from build123d import *

# Parameters (mm, degrees)
BOSS_EXTRUDE1_DEPTH = 3
SKETCH2_R           = 0.75
BOSS_EXTRUDE2_DEPTH = 3
SKETCH3_R           = 2.5
BOSS_EXTRUDE3_DEPTH = 0.5
SKETCH4_R           = 2
BOSS_EXTRUDE4_DEPTH = 2.5


with BuildPart() as part:
    # Sketch1 → Boss-Extrude1 (new body)
    with BuildSketch(Plane(origin=(0, 0, 0), x_dir=(1, 0, 0), z_dir=(0, 1, 0))):
        with BuildLine():
            ThreePointArc((0.59835355, 4.007919609), (0.660413192, 4.106024801), (0.773897857, 4.130463677))
            ThreePointArc((0.773897857, 4.130463677), (0.935108267, 4.096977009), (1.094883149, 4.057200879))
            ThreePointArc((1.094883149, 4.057200879), (1.186525668, 3.985943061), (1.199873226, 3.870626668))
            ThreePointArc((1.199873226, 3.870626668), (1.497913497, 3.110449426), (2.278069066, 3.351394917))
            ThreePointArc((2.278069066, 3.351394917), (2.376549119, 3.412857971), (2.4893989, 3.385637488))
            ThreePointArc((2.4893989, 3.385637488), (2.62011514, 3.285520466), (2.746809119, 3.180359688))
            ThreePointArc((2.746809119, 3.180359688), (2.798458567, 3.076396414), (2.760450393, 2.966708646))
            ThreePointArc((2.760450393, 2.966708646), (2.699146854, 2.152497789), (3.506585066, 2.03108536))
            ThreePointArc((3.506585066, 2.03108536), (3.621980347, 2.043732765), (3.711843962, 1.970244271))
            ThreePointArc((3.711843962, 1.970244271), (3.786176077, 1.823326301), (3.854695856, 1.673609257))
            ThreePointArc((3.854695856, 1.673609257), (3.856122426, 1.557531728), (3.774286506, 1.475197592))
            ThreePointArc((3.774286506, 1.475197592), (3.365781075, 0.768217567), (4.040578887, 0.308494438))
            ThreePointArc((4.040578887, 0.308494438), (4.150033947, 0.269821219), (4.199112803, 0.164620014))
            ThreePointArc((4.199112803, 0.164620014), (4.202338407, 0), (4.199112803, -0.164620014))
            ThreePointArc((4.199112803, -0.164620014), (4.150033947, -0.269821219), (4.040578887, -0.308494438))
            ThreePointArc((4.040578887, -0.308494438), (3.365781075, -0.768217567), (3.774286506, -1.475197592))
            ThreePointArc((3.774286506, -1.475197592), (3.856122426, -1.557531728), (3.854695856, -1.673609257))
            ThreePointArc((3.854695856, -1.673609257), (3.786176077, -1.823326301), (3.711843962, -1.970244271))
            ThreePointArc((3.711843962, -1.970244271), (3.621980347, -2.043732765), (3.506585066, -2.03108536))
            ThreePointArc((3.506585066, -2.03108536), (2.699146854, -2.152497789), (2.760450393, -2.966708646))
            ThreePointArc((2.760450393, -2.966708646), (2.798458567, -3.076396414), (2.746809119, -3.180359688))
            ThreePointArc((2.746809119, -3.180359688), (2.62011514, -3.285520466), (2.4893989, -3.385637488))
            ThreePointArc((2.4893989, -3.385637488), (2.376549119, -3.412857971), (2.278069066, -3.351394917))
            ThreePointArc((2.278069066, -3.351394917), (1.497913497, -3.110449426), (1.199873226, -3.870626668))
            ThreePointArc((1.199873226, -3.870626668), (1.186525668, -3.985943061), (1.094883149, -4.057200879))
            ThreePointArc((1.094883149, -4.057200879), (0.935108267, -4.096977009), (0.773897857, -4.130463677))
            ThreePointArc((0.773897857, -4.130463677), (0.660413192, -4.106024801), (0.59835355, -4.007919609))
            ThreePointArc((0.59835355, -4.007919609), (0, -3.452338407), (-0.59835355, -4.007919609))
            ThreePointArc((-0.59835355, -4.007919609), (-0.660413192, -4.106024801), (-0.773897857, -4.130463677))
            ThreePointArc((-0.773897857, -4.130463677), (-0.935108267, -4.096977009), (-1.094883149, -4.057200879))
            ThreePointArc((-1.094883149, -4.057200879), (-1.186525668, -3.985943061), (-1.199873226, -3.870626668))
            ThreePointArc((-1.199873226, -3.870626668), (-1.497913497, -3.110449426), (-2.278069066, -3.351394917))
            ThreePointArc((-2.278069066, -3.351394917), (-2.376549119, -3.412857971), (-2.4893989, -3.385637488))
            ThreePointArc((-2.4893989, -3.385637488), (-2.62011514, -3.285520466), (-2.746809119, -3.180359688))
            ThreePointArc((-2.746809119, -3.180359688), (-2.798458567, -3.076396414), (-2.760450393, -2.966708646))
            ThreePointArc((-2.760450393, -2.966708646), (-2.699146854, -2.152497789), (-3.506585066, -2.03108536))
            ThreePointArc((-3.506585066, -2.03108536), (-3.621980347, -2.043732765), (-3.711843962, -1.970244271))
            ThreePointArc((-3.711843962, -1.970244271), (-3.786176077, -1.823326301), (-3.854695856, -1.673609257))
            ThreePointArc((-3.854695856, -1.673609257), (-3.856122426, -1.557531728), (-3.774286506, -1.475197592))
            ThreePointArc((-3.774286506, -1.475197592), (-3.365781075, -0.768217567), (-4.040578887, -0.308494438))
            ThreePointArc((-4.040578887, -0.308494438), (-4.150033947, -0.269821219), (-4.199112803, -0.164620014))
            ThreePointArc((-4.199112803, -0.164620014), (-4.202338407, 0), (-4.199112803, 0.164620014))
            ThreePointArc((-4.199112803, 0.164620014), (-4.150033947, 0.269821219), (-4.040578887, 0.308494438))
            ThreePointArc((-4.040578887, 0.308494438), (-3.365781075, 0.768217567), (-3.774286506, 1.475197592))
            ThreePointArc((-3.774286506, 1.475197592), (-3.856122426, 1.557531728), (-3.854695856, 1.673609257))
            ThreePointArc((-3.854695856, 1.673609257), (-3.786176077, 1.823326301), (-3.711843962, 1.970244271))
            ThreePointArc((-3.711843962, 1.970244271), (-3.621980347, 2.043732765), (-3.506585066, 2.03108536))
            ThreePointArc((-3.506585066, 2.03108536), (-2.699146854, 2.152497789), (-2.760450393, 2.966708646))
            ThreePointArc((-2.760450393, 2.966708646), (-2.798458567, 3.076396414), (-2.746809119, 3.180359688))
            ThreePointArc((-2.746809119, 3.180359688), (-2.62011514, 3.285520466), (-2.4893989, 3.385637488))
            ThreePointArc((-2.4893989, 3.385637488), (-2.376549119, 3.412857971), (-2.278069066, 3.351394917))
            ThreePointArc((-2.278069066, 3.351394917), (-1.497913497, 3.110449426), (-1.199873226, 3.870626668))
            ThreePointArc((-1.199873226, 3.870626668), (-1.186525668, 3.985943061), (-1.094883149, 4.057200879))
            ThreePointArc((-1.094883149, 4.057200879), (-0.935108267, 4.096977009), (-0.773897857, 4.130463677))
            ThreePointArc((-0.773897857, 4.130463677), (-0.660413192, 4.106024801), (-0.59835355, 4.007919609))
            ThreePointArc((-0.59835355, 4.007919609), (0, 3.452338407), (0.59835355, 4.007919609))
        make_face()
    extrude(amount=BOSS_EXTRUDE1_DEPTH)

    # Sketch2 → Boss-Extrude2 (add)
    with BuildSketch(Plane(origin=(0, 0, 0), x_dir=(-1, 0, 0), z_dir=(0, -1, 0))):
        with Locations(Location((0, 0, 0), (0, 0, 270))):
            Circle(SKETCH2_R)
    extrude(amount=BOSS_EXTRUDE2_DEPTH)

    # Sketch3 → Boss-Extrude3 (add)
    with BuildSketch(Plane(origin=(0, 3, 0), x_dir=(1, 0, 0), z_dir=(0, 1, 0))):
        with Locations(Location((0, 0, 0), (0, 0, 270))):
            Circle(SKETCH3_R)
    extrude(amount=BOSS_EXTRUDE3_DEPTH)

    # Sketch4 → Boss-Extrude4 (add)
    with BuildSketch(Plane(origin=(0, 3.5, 0), x_dir=(1, 0, 0), z_dir=(0, 1, 0))):
        with Locations(Location((0, 0, 0), (0, 0, 270))):
            Circle(SKETCH4_R)
    extrude(amount=BOSS_EXTRUDE4_DEPTH)


solid = part.part
Could you check a few things on this model? Use its own coordinates, in mm. A direction names the side the tool comes from. Coordinates: 2 decimals unless noted, no trailing zeros. Write each loop counter-clockwise with the first axis right and the second up, starting at its lowest first coordinate (ties: lowest second). Pieces come first, ordered by that corner, then holes. Notation, with made-up numbers: (80.5, 50) - (104.5, 50) arc R21 ccw to (104.5, 73) - close; hole circle Ø6 at (-27, -11). An arc over 180 degrees is marked (long way). Put each result on its own line as item: value. Start each with the question number.
Q1. Please list where these lines run through material, in increasing order: L1, parallel to Y at x = -0.5, z = -3.5; L2, parallel to X at y = -1.5, z = 0; L3, parallel to X at y = 1.75, z = 2.
Q2. I'm going to push flat-ended pins straight in: P1, Ø3, axis at x = 3, z = 3.5, coming from the +Y side; P2, Ø3, axis at y = 5, z = 3, coming from the +X side; P3, Ø2, axis at x = -3.5, y = -0.5, coming from the +Z side. Where does each tip first touch, or does it pass through?
Q3. Thinking about a two-plate mould opening in Z: for faces 4 (the cylindrical face through (-3.369, 1.479, -0.756)), 5 (the flat face through (-2, 3, 2)), 6 (the cylindrical face through (-0.013, 1.479, -3.452)), which applies, pulls with the +Z half, pulls with the -Z half, needs draft (parallel to the pull), parting line crosses it, or undercut?
Q4. I want a section at B-B on x = 0. Write out the boundary of the cut face in (y, z).
Q5. I want a section at C-C on z = 3.75. Write out the boundary of the cut face in (x, y), plus the area to 3 significant figures.
Q6. Which directions (+Z, -Z, +X, -X, +Y, -Y) give clear straight access to the entire face, cutting with the end or side of a thin tool? Please do faces 1 (the flat face through (0, 6, 0)), 2 (the cylindrical face through (-2.44, 3.25, -0.54)), 3 (the cylindrical face through (-0.225, -1.479, 0.715)).
Q7. I want a section at A-A on z = 0. Write out the boundary of the cut face in (x, y).
Q8. I want a section at D-D on y = 5. Write out the boundary of the cut face in (x, z).
Checks:
1. L1: 0 to 3
1. L2: -0.75 to 0.75
1. L3: -3.69 to -3.46, -2.88 to 2.88, 3.46 to 3.69
2. P1: y = 3
2. P2: x = 1.32
2. P3: z = 3.27
3. face 4: undercut
3. face 5: needs draft
3. face 6: pulls with the -Z half
4. outline: (-3, -0.75) - (0, -0.75) - (0, -3.45) - (3, -3.45) - (3, -2.5) - (3.5, -2.5) - (3.5, -2) - (6, -2) - (6, 2) - (3.5, 2) - (3.5, 2.5) - (3, 2.5) - (3, 3.45) - (0, 3.45) - (0, 0.75) - (-3, 0.75) - close
5. outline: (-1.17, 0) - (-0.52, 0) - (-0.52, 3) - (-1.17, 3) - close; (0.52, 0) - (1.17, 0) - (1.17, 3) - (0.52, 3) - close
5. area: 3.89 mm²
6. face 1: +Z, -Z, +X, -X, +Y
6. face 2: +Y
6. face 3: -Y
7. outline: (-4.2, 0) - (-0.75, 0) - (-0.75, -3) - (0.75, -3) - (0.75, 0) - (4.2, 0) - (4.2, 3) - (2.5, 3) - (2.5, 3.5) - (2, 3.5) - (2, 6) - (-2, 6) - (-2, 3.5) - (-2.5, 3.5) - (-2.5, 3) - (-4.2, 3) - close
8. outline: circle Ø4 at (0, 0)
